Geometry: final body of the model. Coordinates: model frame, mm. A direction names the side the tool comes from. Round coordinates to 2 decimals unless told otherwise and drop trailing zeros. Write each loop counter-clockwise with the first axis right and the second up, starting at its lowest first coordinate (ties: lowest second). Pieces come first, ordered by that corner, then holes. Notation, with made-up numbers: (18.5, -26) - (62.5, -26) arc R21 cw to (62.5, 5) - close; hole circle Ø5 at (52, 50.5). An arc over 180 degrees is marked (long way). Use a Markdown table: item, result. Add a question column.
```python
from build123d import *

# Parameters (mm, degrees)
SKETCH_1_W          = 27
SKETCH_1_H          = 11
EXTRUDE_1_DEPTH     = 12
SKETCH_2_W          = 23
SKETCH_2_H          = 7
CUT_EXTRUDE_1_DEPTH = 8
SKETCH_3_W          = 21
SKETCH_3_H          = 5.5
EXTRUDE_2_DEPTH     = 8
SKETCH_4_W          = 9
SKETCH_4_H          = 3
CUT_EXTRUDE_2_DEPTH = 4
SKETCH_5_W          = 1
SKETCH_5_H          = 4
CUT_EXTRUDE_3_DEPTH = 1
EXTRUDE_3_DEPTH     = 3.5
EXTRUDE_4_DEPTH     = 10
CUT_EXTRUDE_4_DEPTH = 0.5
SKETCH_9_W          = 0.2
SKETCH_9_H          = 3.5
EXTRUDE_5_DEPTH     = 0.1
SKETCH_10_W         = 39.75
SKETCH_10_H         = 10
EXTRUDE_6_DEPTH     = 72


with BuildPart() as part:
    # 草图1 → 凸台-拉伸1 (new body)
    with BuildSketch(Plane.XY):
        Rectangle(SKETCH_1_W, SKETCH_1_H)
    extrude(amount=EXTRUDE_1_DEPTH)

    # 草图2 → 切除-拉伸1 (cut)
    with BuildSketch(Plane.XY.offset(12)):
        Rectangle(SKETCH_2_W, SKETCH_2_H)
    extrude(amount=-CUT_EXTRUDE_1_DEPTH, mode=Mode.SUBTRACT)

    # 草图3 → 凸台-拉伸2 (add)
    with BuildSketch(Plane.XY.offset(4)):
        Rectangle(SKETCH_3_W, SKETCH_3_H)
    extrude(amount=EXTRUDE_2_DEPTH)

    # 草图4 → 切除-拉伸2 (cut)
    with BuildSketch(Plane.XY.offset(12)):
        with Locations((5.5, 0)):
            Rectangle(SKETCH_4_W, SKETCH_4_H)
        with Locations((-5.5, 0)):
            Rectangle(SKETCH_4_W, SKETCH_4_H)
    extrude(amount=-CUT_EXTRUDE_2_DEPTH, mode=Mode.SUBTRACT)

    # 草图5 → 切除-拉伸3 (cut)
    with BuildSketch(Plane.XY.offset(12)):
        Rectangle(SKETCH_5_W, SKETCH_5_H)
    extrude(amount=-CUT_EXTRUDE_3_DEPTH, mode=Mode.SUBTRACT)

    # 草图6 → 凸台-拉伸3 (add)
    with BuildSketch(Plane.XY.offset(8)):
        with BuildLine():
            Line((-7.5, -1.5), (-9.5, -1.5))
            ThreePointArc((-9.5, -1.5), (-8.5, -1.085786438), (-7.5, -1.5))
        make_face()
        with BuildLine():
            Line((-4.5, -1.5), (-6.5, -1.5))
            ThreePointArc((-6.5, -1.5), (-5.5, -1.085786438), (-4.5, -1.5))
        make_face()
        with BuildLine():
            Line((-3.5, -1.5), (-1.5, -1.5))
            ThreePointArc((-1.5, -1.5), (-2.5, -1.085786438), (-3.5, -1.5))
        make_face()
        with BuildLine():
            Line((3.5, -1.5), (1.5, -1.5))
            ThreePointArc((1.5, -1.5), (2.5, -1.085786438), (3.5, -1.5))
        make_face()
        with BuildLine():
            Line((4.5, -1.5), (6.5, -1.5))
            ThreePointArc((6.5, -1.5), (5.5, -1.085786438), (4.5, -1.5))
        make_face()
        with BuildLine():
            Line((7.5, -1.5), (9.5, -1.5))
            ThreePointArc((9.5, -1.5), (8.5, -1.085786438), (7.5, -1.5))
        make_face()
    extrude(amount=EXTRUDE_3_DEPTH)

    # 草图7 → 凸台-拉伸4 (add)
    with BuildSketch(Plane(origin=(0, 0, 0), x_dir=(-1, 0, 0), z_dir=(0, 0, -1))):
        with BuildLine():
            Line((-14, -6), (25, -6))
            ThreePointArc((25, -6), (25.353553391, -5.853553391), (25.5, -5.5))
            Line((25.5, -5.5), (25.5, 5.5))
            ThreePointArc((25.5, 5.5), (25.353553391, 5.853553391), (25, 6))
            Line((25, 6), (-14, 6))
            ThreePointArc((-14, 6), (-14.353553391, 5.853553391), (-14.5, 5.5))
            Line((-14.5, 5.5), (-14.5, -5.5))
            ThreePointArc((-14.5, -5.5), (-14.353553391, -5.853553391), (-14, -6))
        make_face()
    extrude(amount=EXTRUDE_4_DEPTH)

    # 草图8 → 切除-拉伸4 (cut)
    with BuildSketch(Plane.XY):
        with BuildLine():
            Line((-23, 1.75), (-16, 1.75))
            ThreePointArc((-16, 1.75), (-14.25, 0), (-16, -1.75))
            Line((-16, -1.75), (-23, -1.75))
            ThreePointArc((-23, -1.75), (-24.75, 0), (-23, 1.75))
        make_face()
    extrude(amount=-CUT_EXTRUDE_4_DEPTH, mode=Mode.SUBTRACT)

    # 草图9 → 凸台-拉伸5 (add)
    with BuildSketch(Plane.XY.offset(-0.5)):
        with Locations((-19.5, 0)):
            Rectangle(SKETCH_9_W, SKETCH_9_H)
    extrude(amount=EXTRUDE_5_DEPTH)

    # 草图10 → 凸台-拉伸6 (add)
    with BuildSketch(Plane.XZ.offset(-6)):
        with Locations((-5.375, -5)):
            Rectangle(SKETCH_10_W, SKETCH_10_H)
    extrude(amount=-EXTRUDE_6_DEPTH)


solid = part.part
```
1) Section B-B, the plane z = 1.25. Return the cut outline in (x, y).
2) Set-up query: faces 1 (the flat face through (13.5, 0, 6)), 2 (the flat face through (0, 3.5, 8)), 3 (the flat face through (-13.5, 0, 6)), 4 (the flat face through (-25.25, 41, -5)). Return all of +Z, -Z, +X, -X, +Y, -Y with unobstructed straight access to the full face (end or side cutting, diameter ignored); none if empty.
3) Section C-C, the plane y = 7. Return the cut outline in (x, z).
4) Material intervals for L1, parallel to Y at x = 2.5, z = 8.25; L2, parallel to Z at x = -19, y = 21.5; L3, parallel to Y at x = 3.5, z = 2.5, sorted ascending. Write a range as from..to.
5) Pin query (flat end, axial travel): P1, Ø1.1, axis at x = 0, z = 11.5, coming from the +Y side; P2, Ø2, axis at y = 66, z = -6, coming from the -X side; P3, Ø0.9, axis at y = 0.5, z = 11, coming from the -X side; P4, Ø12, axis at y = 41, z = 8, coming from the +X side. Return the tip coordinate at first contact, or that it passes through.
6) Section A-A, the plane x = 12.5. Return the cut outline in (y, z).
7) Draft query along Y for faces 5 (the flat face through (-25.5, 0, -5)), 6 (the flat face through (-10.5, 0, 8)), 7 (the flat face through (0, -5.5, 6)). Return one class per face: released by +Y, released by -Y, zero draft, split by the parting line, or undercut.
Output values:
| question | item | result |
|---|---|---|
| 1 | outline | (-13.5, -5.5) - (13.5, -5.5) - (13.5, 5.5) - (-13.5, 5.5) - close |
| 2 | face 1 | +Z, +X, +Y, -Y |
| 2 | face 2 | +Z |
| 2 | face 3 | +Z, -X, +Y, -Y |
| 2 | face 4 | +Z, -Z, -X, +Y |
| 3 | outline | (-25.25, -10) - (14.5, -10) - (14.5, 0) - (-25.25, 0) - close |
| 4 | L1 | y = -5.5..-3.5, -2.75..-1.09, 1.5..2.75, 3.5..5.5 |
| 4 | L2 | z = -10..0 |
| 4 | L3 | y = -5.5..5.5 |
| 5 | P1 | stops at y = 5.5 |
| 5 | P2 | stops at x = -25.25 |
| 5 | P3 | stops at x = -13.5 |
| 5 | P4 | passes through |
| 6 | outline | (-6, -10) - (78, -10) - (78, 0) - (5.5, 0) - (5.5, 12) - (-5.5, 12) - (-5.5, 0) - (-6, 0) - close |
| 7 | face 5 | zero draft |
| 7 | face 6 | undercut |
| 7 | face 7 | released by -Y |
